Could you check a few things on this model? Use its own coordinates, in mm. A direction names the side the tool comes from. Give positions to 0.01 mm unless a question says otherwise; leave off trailing zeros. Loops run counter-clockwise (first coordinate to the right, second up) from the corner with the lowest first, then second, coordinate; pieces in that order, holes last. Notation, with made-up numbers: M 24.25,35 L 49.25,35 A18 ccw 49.25,55 Z; hole C -12.5,21.25 d1. An arc over 180 degrees is marked long. Return JSON: item names as keys, results as strings. Group by question number.
1. If we section it at A-A (x = 0): Write out the boundary of the cut face in (y, z).
2. If we mould it in two halves opening along Y, with no side actions, what happens to faces 1 (the cylindrical face through (-1.01, 13.49, -0.65)), 2 (the flat face through (-1.08, 15.81, -0.63)), 3 (the flat face through (0, 0, 0)), 4 (the flat face through (0, 14.8, 0))? For each: +Y half, -Y half, draft (parallel to the pull), parting line (faces both ways), or undercut.
3. Please list where these lines run through material, in increasing order: line 1 (Y direction, x = 1.05, z = -0.95); line 2 (Y direction, x = 0.45, z = -1.9); line 3 (Z direction, x = 0.4, y = 8).
4. For faces 5 (the cylindrical face through (-0.45, 6.41, -1.43)), 6 (the flat face through (1.088, 15.814, -0.616)), 7 (the flat face through (1.03, 16.8, 1.03)), which set-ups out of +Z, -Z, +X, -X, +Y, -Y let a thin tool reach every point of the face, with its end or its side?
5. If we section it at B-B (y = 6.5): Write out the boundary of the cut face in (x, z).
6. For pin 1 (0.9 mm diameter, centred on x = -0.5, z = 0, fed in from +Y); pin 2 (1.5 mm diameter, centred on y = 10, z = -1, fed in from -X); pin 3 (2 mm diameter, centred on y = 2.5, z = -2, fed in from +X), each with a flat end and sliding along its axis, tell me the tip position at first contact or that it passes through.
```python
from build123d import *

# Parameters (mm, degrees)
CUT_EXTRUDE_1_DEPTH = 2


with BuildPart() as part:
    # 草图1 → 旋转1 (revolve)
    with BuildSketch(Plane.XY, mode=Mode.PRIVATE) as revolve_1_sk:
        with BuildLine():
            Line((0, 16.8), (-2.4, 16.8))
            ThreePointArc((-2.4, 16.8), (-2.682842712, 16.682842712), (-2.8, 16.4))
            Line((-2.8, 16.4), (-2.8, 14.4))
            ThreePointArc((-2.8, 14.4), (-2.682842712, 14.117157288), (-2.4, 14))
            Line((-2.4, 14), (-1.2, 14))
            Line((-1.2, 14), (-1.2, 13))
            Line((-1.2, 13), (-1.5, 13))
            Line((-1.5, 13), (-1.5, 0))
            Line((-1.5, 0), (0, 0))
            Line((0, 0), (0, 16.8))
        make_face()
    revolve(revolve_1_sk.sketch.rotate(Axis((0, 0, 0), (0, 1, 0)), 270), axis=Axis((0, 0, 0), (0, 1, 0)))

    # 草图2 → 切除-拉伸1 (cut)
    with BuildSketch(Plane(origin=(0, 16.8, 0), x_dir=(1, 0, 0), z_dir=(0, 1, 0))):
        Polygon((-0.721687836, 1.25), (-1.443375673, 0), (-0.721687836, -1.25), (0.721687836, -1.25), (1.443375673, 0), (0.721687836, 1.25), align=None)
    extrude(amount=-CUT_EXTRUDE_1_DEPTH, mode=Mode.SUBTRACT)


solid = part.part
```
Answer:
{
 "1": {"outline": "M 0,-1.5 L 13,-1.5 L 13,-1.2 L 14,-1.2 L 14,-2.4 A0.4 ccw 14.4,-2.8 L 16.4,-2.8 A0.4 ccw 16.8,-2.4 L 16.8,-1.25 L 14.8,-1.25 L 14.8,1.25 L 16.8,1.25 L 16.8,2.4 A0.4 ccw 16.4,2.8 L 14.4,2.8 A0.4 ccw 14,2.4 L 14,1.2 L 13,1.2 L 13,1.5 L 0,1.5 Z"},
 "2": {"face 1": "undercut", "face 2": "draft", "face 3": "-Y half", "face 4": "+Y half"},
 "3": {"line 1": "y = 0 to 13, 14 to 16.8", "line 2": "y = 14 to 16.8", "line 3": "z = -1.45 to 1.45"},
 "4": {"face 5": "-Y", "face 6": "+Y", "face 7": "+Z, -Z, +X, -X, +Y"},
 "5": {"outline": "C 0,0 d3"},
 "6": {"pin 1": "stops at y = 14.8", "pin 2": "stops at x = -1.48", "pin 3": "stops at x = 1.12"}
}
